Part model, mm, in its own coordinate system. A direction names the side the tool comes from. Coordinates: 2 decimals unless noted, no trailing zeros. Loops run counter-clockwise (first coordinate to the right, second up) from the corner with the lowest first, then second, coordinate; pieces in that order, holes last. Notation, with made-up numbers: (-35.75, -1.5) - (-10.75, -1.5) arc R20 ccw to (-10.75, 17.5) - close; hole circle Ø5 at (7, 32). An arc over 180 degrees is marked (long way). Use a Markdown table: item, result. Add a question column.
1. Wall check: probe 1 along X at (y, z) = (1.4, 8); probe 2 along Z at (x, y) = (24.5, 2.7); probe 3 along Z at (x, y) = (80, 1.45). Give the ranges that are in metal, low to high. Write a range as [from, to].
2. Band-saw the part on A-A, the plane x = -7.5. Give the cut face in (y, z), plus the area to 3 significant figures.
3. Band-saw the part on B-B, the plane z = -8. Give the cut face in (x, y).
4. Band-saw the part on D-D, the plane x = -75. Give the cut face in (y, z).
5. 3-axis set-ups, long thin cutter, end or side, ignore diameter. For faces 1 (the cylindrical face through (-83.57, 1.48, -41)), 2 (the flat face through (7, 2, 3.8)): which of +Z, -Z, +X, -X, +Y, -Y reach the whole face in a straight line?
6. Band-saw the part on C-C, the plane x = 28. Give the cut face in (y, z), plus the area to 3 significant figures.
7. Pull direction X, two halves, no side cores. Call faces 3 (the cylindrical face through (83.5, 1.48, -41.07)), 4 (the cylindrical face through (-83.5, 1.48, 41.07)), 5 (the cylindrical face through (-62.586, 1.479, -7.792)): pulls with the +X half, pulls with the -X half, needs draft (parallel to the pull), parting line crosses it, or undercut.
from build123d import *

# Parameters (mm, degrees)
SKETCH1_R           = 1.6
BOSS_EXTRUDE1_DEPTH = 3
CUT_EXTRUDE1_DEPTH  = 3
SKETCH3_R           = 1.6
CUT_EXTRUDE2_DEPTH  = 3


with BuildPart() as part:
    # Sketch1 → Boss-Extrude1 (new body)
    with BuildSketch(Plane(origin=(0, 0, 0), x_dir=(1, 0, 0), z_dir=(0, 1, 0))):
        with BuildLine():
            Line((-80, 42.5), (80, 42.5))
            ThreePointArc((80, 42.5), (83.535533906, 41.035533906), (85, 37.5))
            Line((85, 37.5), (85, -37.5))
            ThreePointArc((85, -37.5), (83.535533906, -41.035533906), (80, -42.5))
            Line((80, -42.5), (-80, -42.5))
            ThreePointArc((-80, -42.5), (-83.535533906, -41.035533906), (-85, -37.5))
            Line((-85, -37.5), (-85, 37.5))
            ThreePointArc((-85, 37.5), (-83.535533906, 41.035533906), (-80, 42.5))
        make_face()
        with Locations(Location((-80, 37.5, 0), (0, 0, 270))):
            Circle(SKETCH1_R, mode=Mode.SUBTRACT)
        with Locations(Location((80, 37.5, 0), (0, 0, 270))):
            Circle(SKETCH1_R, mode=Mode.SUBTRACT)
        with Locations(Location((-80, -37.5, 0), (0, 0, 270))):
            Circle(SKETCH1_R, mode=Mode.SUBTRACT)
        with Locations(Location((80, -37.5, 0), (0, 0, 270))):
            Circle(SKETCH1_R, mode=Mode.SUBTRACT)
        with Locations(Location((-75, 8, 0), (0, 0, 270))):
            Circle(SKETCH1_R, mode=Mode.SUBTRACT)
        with Locations(Location((-75, -8, 0), (0, 0, 90))):
            Circle(SKETCH1_R, mode=Mode.SUBTRACT)
        with Locations(Location((-61, -8, 0), (0, 0, 270))):
            Circle(SKETCH1_R, mode=Mode.SUBTRACT)
        with Locations(Location((-61, 8, 0), (0, 0, 90))):
            Circle(SKETCH1_R, mode=Mode.SUBTRACT)
        with Locations(Location((61, -8, 0), (0, 0, 90))):
            Circle(SKETCH1_R, mode=Mode.SUBTRACT)
        with Locations(Location((75, -8, 0), (0, 0, 270))):
            Circle(SKETCH1_R, mode=Mode.SUBTRACT)
        with Locations(Location((61, 8, 0), (0, 0, 270))):
            Circle(SKETCH1_R, mode=Mode.SUBTRACT)
        with Locations(Location((75, 8, 0), (0, 0, 90))):
            Circle(SKETCH1_R, mode=Mode.SUBTRACT)
        with Locations(Location((-50.75, 20, 0), (0, 0, 270))):
            Circle(SKETCH1_R, mode=Mode.SUBTRACT)
        with Locations(Location((-10.75, 20, 0), (0, 0, 90))):
            Circle(SKETCH1_R, mode=Mode.SUBTRACT)
        with Locations(Location((-10.75, -20, 0), (0, 0, 270))):
            Circle(SKETCH1_R, mode=Mode.SUBTRACT)
        with Locations(Location((-50.75, -20, 0), (0, 0, 90))):
            Circle(SKETCH1_R, mode=Mode.SUBTRACT)
        with Locations(Location((50.75, -20, 0), (0, 0, 270))):
            Circle(SKETCH1_R, mode=Mode.SUBTRACT)
        with Locations(Location((10.75, -20, 0), (0, 0, 90))):
            Circle(SKETCH1_R, mode=Mode.SUBTRACT)
        with Locations(Location((10.75, 20, 0), (0, 0, 270))):
            Circle(SKETCH1_R, mode=Mode.SUBTRACT)
        with Locations(Location((50.75, 20, 0), (0, 0, 90))):
            Circle(SKETCH1_R, mode=Mode.SUBTRACT)
        with Locations(Location((0, 19.68, 0), (0, 0, 270))):
            Circle(SKETCH1_R, mode=Mode.SUBTRACT)
        with Locations(Location((0, -19.68, 0), (0, 0, 90))):
            Circle(SKETCH1_R, mode=Mode.SUBTRACT)
        with BuildLine():
            Line((-38, 38.5), (38, 38.5))
            ThreePointArc((38, 38.5), (39.414213562, 37.914213562), (40, 36.5))
            Line((40, 36.5), (40, 32.5))
            ThreePointArc((40, 32.5), (39.414213562, 31.085786438), (38, 30.5))
            Line((38, 30.5), (-38, 30.5))
            ThreePointArc((-38, 30.5), (-39.414213562, 31.085786438), (-40, 32.5))
            Line((-40, 32.5), (-40, 36.5))
            ThreePointArc((-40, 36.5), (-39.414213562, 37.914213562), (-38, 38.5))
        make_face(mode=Mode.SUBTRACT)
        with BuildLine():
            Line((40, -36.5), (40, -32.5))
            ThreePointArc((40, -32.5), (39.414213562, -31.085786438), (38, -30.5))
            Line((38, -30.5), (-38, -30.5))
            ThreePointArc((-38, -30.5), (-39.414213562, -31.085786438), (-40, -32.5))
            Line((-40, -32.5), (-40, -36.5))
            ThreePointArc((-40, -36.5), (-39.414213562, -37.914213562), (-38, -38.5))
            Line((-38, -38.5), (38, -38.5))
            ThreePointArc((38, -38.5), (39.414213562, -37.914213562), (40, -36.5))
        make_face(mode=Mode.SUBTRACT)
    extrude(amount=BOSS_EXTRUDE1_DEPTH)

    # Sketch2 → Cut-Extrude1 (cut)
    with BuildSketch(Plane(origin=(0, 3, 0), x_dir=(1, 0, 0), z_dir=(0, 1, 0))):
        with BuildLine():
            Line((54.5, 37.05), (65.5, 37.05))
            ThreePointArc((65.5, 37.05), (66.914213562, 36.464213562), (67.5, 35.05))
            Line((67.5, 35.05), (67.5, 29.95))
            ThreePointArc((67.5, 29.95), (66.914213562, 28.535786438), (65.5, 27.95))
            Line((65.5, 27.95), (54.5, 27.95))
            ThreePointArc((54.5, 27.95), (53.085786438, 28.535786438), (52.5, 29.95))
            Line((52.5, 29.95), (52.5, 35.05))
            ThreePointArc((52.5, 35.05), (53.085786438, 36.464213562), (54.5, 37.05))
        make_face()
        with BuildLine():
            Line((67.5, -35.05), (67.5, -29.95))
            ThreePointArc((67.5, -29.95), (66.914213562, -28.535786438), (65.5, -27.95))
            Line((65.5, -27.95), (54.5, -27.95))
            ThreePointArc((54.5, -27.95), (53.085786438, -28.535786438), (52.5, -29.95))
            Line((52.5, -29.95), (52.5, -35.05))
            ThreePointArc((52.5, -35.05), (53.085786438, -36.464213562), (54.5, -37.05))
            Line((54.5, -37.05), (65.5, -37.05))
            ThreePointArc((65.5, -37.05), (66.914213562, -36.464213562), (67.5, -35.05))
        make_face()
        with BuildLine():
            Line((-54.5, -37.05), (-65.5, -37.05))
            ThreePointArc((-65.5, -37.05), (-66.914213562, -36.464213562), (-67.5, -35.05))
            Line((-67.5, -35.05), (-67.5, -29.95))
            ThreePointArc((-67.5, -29.95), (-66.914213562, -28.535786438), (-65.5, -27.95))
            Line((-65.5, -27.95), (-54.5, -27.95))
            ThreePointArc((-54.5, -27.95), (-53.085786438, -28.535786438), (-52.5, -29.95))
            Line((-52.5, -29.95), (-52.5, -35.05))
            ThreePointArc((-52.5, -35.05), (-53.085786438, -36.464213562), (-54.5, -37.05))
        make_face()
        with BuildLine():
            Line((-67.5, 35.05), (-67.5, 29.95))
            ThreePointArc((-67.5, 29.95), (-66.914213562, 28.535786438), (-65.5, 27.95))
            Line((-65.5, 27.95), (-54.5, 27.95))
            ThreePointArc((-54.5, 27.95), (-53.085786438, 28.535786438), (-52.5, 29.95))
            Line((-52.5, 29.95), (-52.5, 35.05))
            ThreePointArc((-52.5, 35.05), (-53.085786438, 36.464213562), (-54.5, 37.05))
            Line((-54.5, 37.05), (-65.5, 37.05))
            ThreePointArc((-65.5, 37.05), (-66.914213562, 36.464213562), (-67.5, 35.05))
        make_face()
    extrude(amount=-CUT_EXTRUDE1_DEPTH, mode=Mode.SUBTRACT)

    # Sketch3 → Cut-Extrude2 (cut)
    with BuildSketch(Plane(origin=(0, 3, 0), x_dir=(1, 0, 0), z_dir=(0, 1, 0))):
        with Locations(Location((-7.5, -5.4, 0), (0, 0, 270))):
            Circle(SKETCH3_R)
        with Locations(Location((17.465, 17.395, 0), (0, 0, 270))):
            Circle(SKETCH3_R)
        with Locations(Location((17.465, -17.395, 0), (0, 0, 90))):
            Circle(SKETCH3_R)
        with Locations(Location((79.945, -17.395, 0), (0, 0, 270))):
            Circle(SKETCH3_R)
        with Locations(Location((79.945, 17.395, 0), (0, 0, 90))):
            Circle(SKETCH3_R)
        with BuildLine():
            Line((4.5, -3.8), (10.5, -3.8))
            ThreePointArc((10.5, -3.8), (12.1, -5.4), (10.5, -7))
            Line((10.5, -7), (4.5, -7))
            ThreePointArc((4.5, -7), (2.9, -5.4), (4.5, -3.8))
        make_face()
        with BuildLine():
            Line((-25.2, 13.8), (-25.2, 19.8))
            ThreePointArc((-25.2, 19.8), (-23.6, 21.4), (-22, 19.8))
            Line((-22, 19.8), (-22, 13.8))
            ThreePointArc((-22, 13.8), (-23.6, 12.2), (-25.2, 13.8))
        make_face()
        with BuildLine():
            Line((-39.4, -21), (-45.4, -21))
            ThreePointArc((-45.4, -21), (-47, -19.4), (-45.4, -17.8))
            Line((-45.4, -17.8), (-39.4, -17.8))
            ThreePointArc((-39.4, -17.8), (-37.8, -19.4), (-39.4, -21))
        make_face()
    extrude(amount=-CUT_EXTRUDE2_DEPTH, mode=Mode.SUBTRACT)


solid = part.part
Geometry check:
| question | item | result |
|---|---|---|
| 1 | probe 1 | x = [-85, -76.6], [-73.4, -62.6], [-59.4, 59.4], [62.6, 73.4], [76.6, 85] |
| 1 | probe 2 | z = [-42.5, -38.5], [-30.5, 30.5], [38.5, 42.5] |
| 1 | probe 3 | z = [-42.5, -39.1], [-35.9, -18.99], [-15.8, 15.8], [18.99, 35.9], [39.1, 42.5] |
| 2 | outline | (0, -42.5) - (3, -42.5) - (3, -38.5) - (0, -38.5) - close; (0, -30.5) - (3, -30.5) - (3, 3.8) - (0, 3.8) - close; (0, 7) - (3, 7) - (3, 30.5) - (0, 30.5) - close; (0, 38.5) - (3, 38.5) - (3, 42.5) - (0, 42.5) - close |
| 2 | area | 197 mm^2 |
| 3 | outline | (-85, 0) - (-76.6, 0) - (-76.6, 3) - (-85, 3) - close; (-73.4, 0) - (-62.6, 0) - (-62.6, 3) - (-73.4, 3) - close; (-59.4, 0) - (59.4, 0) - (59.4, 3) - (-59.4, 3) - close; (62.6, 0) - (73.4, 0) - (73.4, 3) - (62.6, 3) - close; (76.6, 0) - (85, 0) - (85, 3) - (76.6, 3) - close |
| 4 | outline | (0, -42.5) - (3, -42.5) - (3, -9.6) - (0, -9.6) - close; (0, -6.4) - (3, -6.4) - (3, 6.4) - (0, 6.4) - close; (0, 9.6) - (3, 9.6) - (3, 42.5) - (0, 42.5) - close |
| 5 | face 1 | -Z, -X, +Y, -Y |
| 5 | face 2 | +Y, -Y |
| 6 | outline | (0, -42.5) - (3, -42.5) - (3, -38.5) - (0, -38.5) - close; (0, -30.5) - (3, -30.5) - (3, 30.5) - (0, 30.5) - close; (0, 38.5) - (3, 38.5) - (3, 42.5) - (0, 42.5) - close |
| 6 | area | 207 mm^2 |
| 7 | face 3 | pulls with the +X half |
| 7 | face 4 | pulls with the -X half |
| 7 | face 5 | undercut |
